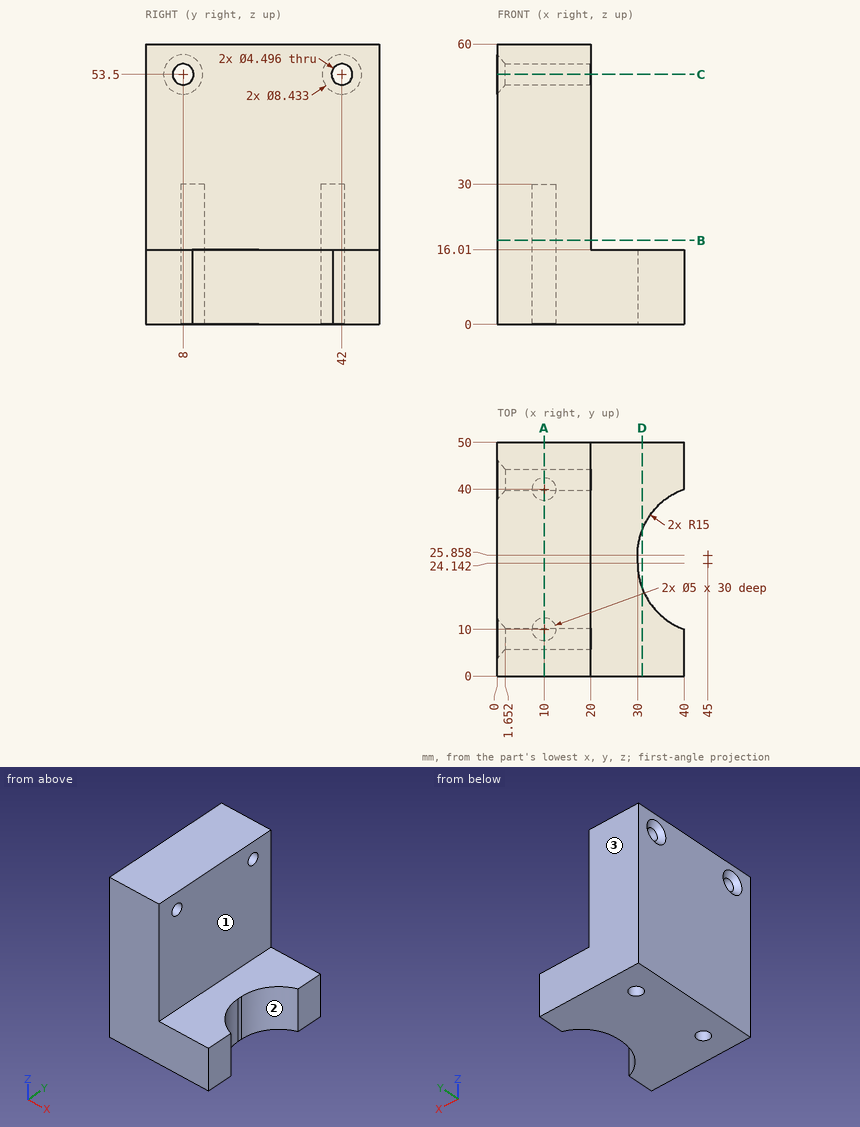
Verification items for this drawing (mm, ordinates from the low corner). A direction names the side the tool comes from. Round coordinates to 2 decimals unless told otherwise and drop trailing zeros. Loops run counter-clockwise (first coordinate to the right, second up) from the corner with the lowest first, then second, coordinate; pieces in that order, holes last. Notation, with made-up numbers: (46.5, 17) -> (69.5, 17) arc R34 ccw to (69.5, 50) -> close; hole circle Ø2 at (21.5, 41.5). An arc over 180 degrees is marked (long way). Answer in a Markdown table with one row per item.
Q1. Thickness scan on L1, parallel to Y at x = 10, z = 9.75; L2, parallel to Y at x = 11.5, z = 55.5 (1 decimal); L3, parallel to Z at x = 23.5, y = 14.5. Record the ranges inside material, lowest first.
Data:
| item | result |
|---|---|
| L1 | y = 0 to 7.5, 12.5 to 37.5, 42.5 to 50 |
| L2 | y = 0 to 7, 9 to 41, 43 to 50 |
| L3 | z = 0 to 16.01 |
Q2. Sectioned sample at B-B on z = 18. Enter the section's corners in (x, y).
Data:
| item | result |
|---|---|
| outline | (0, 0) -> (20, 0) -> (20, 50) -> (0, 50) -> close; hole circle Ø5 at (10, 10); hole circle Ø5 at (10, 40) |
Q3. Sectioned sample at A-A on x = 10. Enter the section's corners in (y, z).
Data:
| item | result |
|---|---|
| outline | (0, 0) -> (7.5, 0) -> (7.5, 30) -> (12.5, 30) -> (12.5, 0) -> (37.5, 0) -> (37.5, 30) -> (42.5, 30) -> (42.5, 0) -> (50, 0) -> (50, 60) -> (0, 60) -> close; hole circle Ø4.5 at (8, 53.5); hole circle Ø4.5 at (42, 53.5) |
Q4. Go/stop test with flat-tipped pins: P1, Ø8, axis at y = 6, z = 53, coming from the +X side; P2, Ø3.5, axis at y = 8, z = 53.5, coming from the -X side; P3, Ø1.5, axis at x = 11, y = 40, coming from the -Z side; P4, Ø6, axis at x = 29.5, y = 22.5, coming from the +Z side. Record where each tip stops, or that it passes through.
Data:
| item | result |
|---|---|
| P1 | stops at x = 20 |
| P2 | passes through |
| P3 | stops at z = 30 |
| P4 | stops at z = 16.01 |
Q5. Sectioned sample at C-C on z = 53.5. Enter the section's corners in (x, y).
Data:
| item | result |
|---|---|
| outline | (0, 0) -> (20, 0) -> (20, 5.75) -> (1.65, 5.75) -> (0, 3.78) -> close; (0, 12.22) -> (1.65, 10.25) -> (20, 10.25) -> (20, 39.75) -> (1.65, 39.75) -> (0, 37.78) -> close; (0, 46.22) -> (1.65, 44.25) -> (20, 44.25) -> (20, 50) -> (0, 50) -> close |
Q6. Set-up check for the marked faces 1, 2 and 3: record each of +Z, -Z, +X, -X, +Y, -Y from which the full face is reachable in a straight line by a thin tool's end or side.
Data:
| item | result |
|---|---|
| face 1 | +Z, +X, +Y, -Y |
| face 2 | +Z, -Z, +X |
| face 3 | +Z, -Z, +X, -X, +Y |
Q7. Sectioned sample at D-D on x = 31. Enter the section's corners in (y, z).
Data:
| item | result |
|---|---|
| outline | (0, 0) -> (18.76, 0) -> (18.76, 16.01) -> (0, 16.01) -> close; (31.24, 0) -> (50, 0) -> (50, 16.01) -> (31.24, 16.01) -> close |
